```python
from build123d import *

# Parameters (mm, degrees)
F0_W     = 25.4
F0_H     = 25.4
F1_DEPTH = 25.4
F2_R     = 1.905
F4_DEPTH = 5.08


with BuildPart() as f1:
    # F0 (on Top) → F1 (new body)
    with BuildSketch(Plane.XY):
        with Locations((0, 0.155061)):
            Rectangle(F0_W, F0_H)
    extrude(amount=F1_DEPTH)

    # F2
    f2_edges = [f1.edges().sort_by_distance(p)[0] for p in [
        (0, 12.855061, 25.4),
        (-12.7, 0.155061, 25.4),
        (0, -12.544939, 25.4),
        (12.7, 0.155061, 25.4),
        (12.7, -12.544939, 12.7),
        (12.7, 12.855061, 12.7),
        (12.7, 0.155061, 0),
        (-12.7, -12.544939, 12.7),
        (0, -12.544939, 0),
        (-12.7, 12.855061, 12.7),
        (0, 12.855061, 0),
        (-12.7, 0.155061, 0),
    ]]
    fillet(f2_edges, radius=F2_R)

    # F3 (on face) → F4 (cut)
    with BuildSketch(Plane(origin=(0, 12.855061, 0), x_dir=(-1, 0, 0), z_dir=(0, 1, 0))):
        Polygon((0.008823, 8.3006), (3.814404, 10.50794), (3.805581, 14.907341), (-0.008823, 17.0994), (-3.814404, 14.89206), (-3.805581, 10.492659), align=None)
    extrude(amount=-F4_DEPTH, mode=Mode.SUBTRACT)


solid = f1.part
```
For this review, take the finished solid that the model builds, in its own axes (mm). A direction names the side the tool comes from. Coordinates: 2 decimals unless noted, no trailing zeros. Loops run counter-clockwise (first coordinate to the right, second up) from the corner with the lowest first, then second, coordinate; pieces in that order, holes last. Notation, with made-up numbers: (41.5, -10.5) - (64.5, -10.5) arc R28 ccw to (64.5, 7.5) - close; hole circle Ø10 at (-1, 83.5). An arc over 180 degrees is marked (long way). Use one line per item in the form item = value. Start each with the question number.
1) Draft analysis for pull direction X (two halves, no side actions). For faces 1 (the face through (12.16, 12.28, 12.85)), 2 (the face through (1.885, 10.351, 16.011)), 3 (the face through (1.925, 10.351, 9.412)), 4 (the face through (-0.2, 12.855, 17.3)), state which applies: released by +X, released by -X, zero draft, split by the parting line, or undercut.
2) Take a section at A-A (y = 8.25). State the section outline as (x, z) points (3 decimals).
3) Take a section at B-B (z = 16). State the section outline as (x, y) points (3 decimals), plus the area to 3 significant figures.
4) Take a section at C-C (x = -1.25). State the section outline as (y, z) points (3 decimals).
5) For faces 5 (the face through (0.15, -12, 24.83)), 6 (the face through (-1.885, 10.351, 9.389)), list the 3-axis set-ups (+Z, -Z, +X, -X, +Y, -Y) from which the entire face can be reached by the end or side of a thin tool; tool diameter is ignored.
6) To check wall thickness, follow probe 1 along Y at (x, z) = (3, 12.5); probe 2 along Y at (x, z) = (3, 1.75); probe 3 along Z at (x, y) = (11, -6). State the ranges of each line that lie inside material, in increasing order. Write a range as from..to.
From the geometry:
q1.face_1 = released by +X
q1.face_2 = undercut
q1.face_3 = undercut
q1.face_4 = zero draft
q2.outline = (-12.7, 1.905) arc R1.905 ccw to (-10.795, 0) - (10.795, 0) arc R1.905 ccw to (12.7, 1.905) - (12.7, 23.495) arc R1.905 ccw to (10.795, 25.4) - (-10.795, 25.4) arc R1.905 ccw to (-12.7, 23.495) - close; hole (-3.814, 10.508) - (-0.009, 8.301) - (3.806, 10.493) - (3.814, 14.892) - (0.009, 17.099) - (-3.806, 14.907) - close
q3.outline = (-12.7, -10.64) arc R1.905 ccw to (-10.795, -12.545) - (10.795, -12.545) arc R1.905 ccw to (12.7, -10.64) - (12.7, 10.95) arc R1.905 ccw to (10.795, 12.855) - (1.904, 12.855) - (1.904, 7.775) - (-1.904, 7.775) - (-1.904, 12.855) - (-10.795, 12.855) arc R1.905 ccw to (-12.7, 10.95) - close
q3.area = 623 mm2
q4.outline = (-12.545, 1.905) arc R1.905 ccw to (-10.64, 0) - (10.95, 0) arc R1.905 ccw to (12.855, 1.905) - (12.855, 9.021) - (7.775, 9.021) - (7.775, 16.376) - (12.855, 16.376) - (12.855, 23.495) arc R1.905 ccw to (10.95, 25.4) - (-10.64, 25.4) arc R1.905 ccw to (-12.545, 23.495) - close
q5.face_5 = +Z, +X, -X, -Y
q5.face_6 = +Y
q6.probe_1 = -12.54..7.78
q6.probe_2 = -12.54..12.85
q6.probe_3 = 0.01..25.39
